The model under review builds one solid part; all positions refer to its coordinate system, in mm. Face numbers are marked on the shaded views. A direction names the side the tool comes from. Round coordinates to 2 decimals unless told otherwise and drop trailing zeros. Order: outer loops, then holes, each group sorted by start corner. A loop starts at its lowest first (then second) coordinate and runs counter-clockwise, first axis right, second up.
from build123d import *

# Parameters (mm, degrees)
F1_DEPTH  = 5
F3_DEPTH  = 80
F4_W      = 16
F4_H      = 15
F4_H_2    = 5
F5_DEPTH  = 20
F7_W      = 16
F7_H      = 15
F7_H_2    = 5
F8_DEPTH  = 20
F10_DEPTH = 16
F11_R     = 6.35
F13_DEPTH = 80
F16_DEPTH = 20
F18_DEPTH = 10


with BuildPart() as f1:
    # F0 (on Top) → F1 (new body)
    with BuildSketch(Plane.XY):
        Polygon((40, 0), (40, 8), (-40, 8), (-40, 0), (-40, -8), (40, -8), align=None)
    extrude(amount=F1_DEPTH)

    # F2 (on face) → F3 (join)
    with BuildSketch(Plane.YZ.offset(40)):
        Polygon((8, 0), (-8, 0), (8, -16), align=None)
    extrude(amount=-F3_DEPTH)

    # F4 (on face) → F5 (join)
    with BuildSketch(Plane.YZ.offset(40)):
        with Locations((0, 12.5)):
            Rectangle(F4_W, F4_H)
        with Locations((0, 2.5)):
            Rectangle(F4_W, F4_H_2)
    extrude(amount=F5_DEPTH)

    # F7 (on face) → F8 (join)
    with BuildSketch(Plane(origin=(-40, 0, 0), x_dir=(0, -1, 0), z_dir=(-1, 0, 0))):
        with Locations((0, 12.5)):
            Rectangle(F7_W, F7_H)
        with Locations((0, 2.5)):
            Rectangle(F7_W, F7_H_2)
    extrude(amount=F8_DEPTH)

    # F9 (on face) + F6 (on face) → F10 (cut)
    with BuildSketch(Plane.XZ.offset(8)):
        with BuildLine():
            ThreePointArc((-44.2724350724, 15.7275649276), (-55.7275649276, 15.7275649276), (-55.7275649276, 4.2724350724))
            Line((-55.7275649276, 4.2724350724), (-50, 10))
            Line((-50, 10), (-44.2724350724, 15.7275649276))
        make_face()
        with BuildLine():
            Line((-50, 10), (-55.7275649276, 4.2724350724))
            ThreePointArc((-55.7275649276, 4.2724350724), (-46.9002641978, 2.5165757867), (-41.9, 10))
            ThreePointArc((-41.9, 10), (-42.5165757867, 13.0997358022), (-44.2724350724, 15.7275649276))
            Line((-44.2724350724, 15.7275649276), (-50, 10))
        make_face()
    with BuildSketch(Plane.XZ.offset(8)):
        with BuildLine():
            ThreePointArc((44.2724350724, 15.7275649276), (44.2724350724, 4.2724350724), (55.7275649276, 4.2724350724))
            Line((55.7275649276, 4.2724350724), (50, 10))
            Line((50, 10), (44.2724350724, 15.7275649276))
        make_face()
        with BuildLine():
            Line((50, 10), (55.7275649276, 4.2724350724))
            ThreePointArc((55.7275649276, 4.2724350724), (57.4834242133, 6.9002641978), (58.1, 10))
            ThreePointArc((58.1, 10), (53.0997358022, 17.4834242133), (44.2724350724, 15.7275649276))
            Line((44.2724350724, 15.7275649276), (50, 10))
        make_face()
    extrude(amount=-F10_DEPTH, mode=Mode.SUBTRACT)

    # F11
    f11_edges = [f1.edges().sort_by_distance(p)[0] for p in [
        (40, 0, 20),
        (60, 0, 20),
        (60, 0, 0),
        (-60, 0, 0),
        (-60, 0, 20),
        (-40, 0, 20),
    ]]
    fillet(f11_edges, radius=F11_R)

    # F12 (on face) → F13 (cut)
    with BuildSketch(Plane.YZ.offset(40)):
        Polygon((8, -16), (8, 0), (-8, 0), align=None)
    extrude(amount=-F13_DEPTH, mode=Mode.SUBTRACT)

    # F14 (on face) + F15 (on face) → F16 (cut)
    with BuildSketch(Plane.XY.offset(20)):
        with BuildLine():
            Line((-50, 0), (-50.6226316309, -1.3646720677))
            ThreePointArc((-50.6226316309, -1.3646720677), (-49.1888118117, -1.2617344107), (-48.5, 0))
            ThreePointArc((-48.5, 0), (-48.7382655893, 0.8111881883), (-49.3773683691, 1.3646720677))
            Line((-49.3773683691, 1.3646720677), (-50, 0))
        make_face()
        with BuildLine():
            ThreePointArc((-49.3773683691, 1.3646720677), (-51.3646720677, 0.6226316309), (-50.6226316309, -1.3646720677))
            Line((-50.6226316309, -1.3646720677), (-50, 0))
            Line((-50, 0), (-49.3773683691, 1.3646720677))
        make_face()
    with BuildSketch(Plane.XY.offset(20)):
        with BuildLine():
            Line((50, 0), (49.3773683691, -1.3646720677))
            ThreePointArc((49.3773683691, -1.3646720677), (50.8111881883, -1.2617344107), (51.5, 0))
            ThreePointArc((51.5, 0), (51.2617344107, 0.8111881883), (50.6226316309, 1.3646720677))
            Line((50.6226316309, 1.3646720677), (50, 0))
        make_face()
        with BuildLine():
            ThreePointArc((50.6226316309, 1.3646720677), (48.6353279323, 0.6226316309), (49.3773683691, -1.3646720677))
            Line((49.3773683691, -1.3646720677), (50, 0))
            Line((50, 0), (50.6226316309, 1.3646720677))
        make_face()
    extrude(amount=-F16_DEPTH, mode=Mode.SUBTRACT)

    # F17 (on face) → F18 (cut)
    with BuildSketch(Plane.XY.offset(5)):
        with BuildLine():
            Line((-22.5, 0), (-24, 0))
            ThreePointArc((-24, 0), (-22.5, -1.5), (-21, 0))
            Line((-21, 0), (-22.5, 0))
        make_face()
        with BuildLine():
            ThreePointArc((-21, 0), (-22.5, 1.5), (-24, 0))
            Line((-24, 0), (-22.5, 0))
            Line((-22.5, 0), (-21, 0))
        make_face()
        with BuildLine():
            Line((22.5, 0), (21, 0))
            ThreePointArc((21, 0), (22.5, -1.5), (24, 0))
            Line((24, 0), (22.5, 0))
        make_face()
        with BuildLine():
            ThreePointArc((24, 0), (22.5, 1.5), (21, 0))
            Line((21, 0), (22.5, 0))
            Line((22.5, 0), (24, 0))
        make_face()
    extrude(amount=-F18_DEPTH, mode=Mode.SUBTRACT)


solid = f1.part
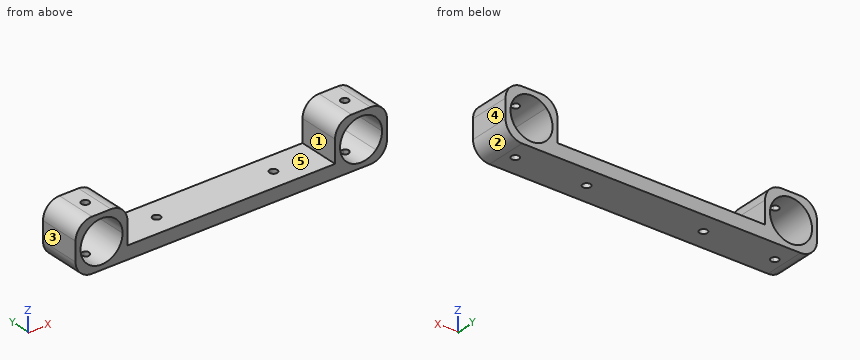
(1) We need section A-A (x = -22.5). Give the boundary of the cut face in (y, z).
(2) Tool access review of the marked faces 4 and 5: name each direction out of +Z, -Z, +X, -X, +Y, -Y from which nothing blocks a thin tool from reaching the whole face with its end or side.
(3) We need section C-C (x = 22). Give the boundary of the cut face in (y, z).
(4) Clearance check with flat-ended pins moving along their axes: P1, Ø1, axis at y = -4.5, z = 5.5, coming from the -X side; P2, Ø12, axis at x = -26, z = 5.5, coming from the -Y side; P3, Ø8, axis at x = -37, y = 5.5, coming from the +Z side; P4, Ø5, axis at x = 31, y = 5, coming from the +Z side. State where each tip first meets the part, or that it passes through.
(5) We need section B-B (y = 4.25). Give the boundary of the cut face in (x, z), and give its area (3 significant figures).
(6) To check wall thickness, follow L1, parallel to X at y = 7.25, z = 9.75; L2, parallel to Y at x = -22.5, z = 2.3; L3, parallel to X at y = 1, z = 15.25. State the ranges of each line that lie inside material, in increasing order.
(7) The part is to be moulded in two halves that separate along X. For the marked faces 1, 2 and 3, say which applies: pulls with the +X half, pulls with the -X half, needs draft (parallel to the pull), parting line crosses it, or undercut.
Verdict:
1. outline: (-8, 0) - (-1.5, 0) - (-1.5, 5) - (-8, 5) - close; (1.5, 0) - (8, 0) - (8, 5) - (1.5, 5) - close
2. face 4: +Z, -Z, +X, +Y, -Y
2. face 5: +Z, +Y, -Y
3. outline: (-8, 0) - (-1.41, 0) - (-1.41, 5) - (-8, 5) - close; (1.41, 0) - (8, 0) - (8, 5) - (1.41, 5) - close
4. P1: stops at x = -59.99
4. P2: stops at y = -8
4. P3: stops at z = 17.07
4. P4: stops at z = 5
5. outline: (-60, 6.35) arc R6.35 ccw to (-53.65, 0) - (53.65, 0) arc R6.35 ccw to (60, 6.35) - (60, 13.65) arc R6.35 ccw to (53.65, 20) - (46.35, 20) arc R6.35 ccw to (40, 13.65) - (40, 5) - (-40, 5) - (-40, 13.65) arc R6.35 ccw to (-46.35, 20) - (-53.65, 20) arc R6.35 ccw to (-60, 13.65) - close; hole circle Ø16.2 at (-50, 10); hole circle Ø16.2 at (50, 10)
5. area: 736 mm2
6. L1: x = -60 to -58.1, -41.9 to -40, 40 to 41.9, 58.1 to 60
6. L2: y = -8 to -1.5, 1.5 to 8
6. L3: x = -59.8 to -56.17, -43.83 to -40.2, 40.2 to 43.83, 56.17 to 59.8
7. face 1: undercut
7. face 2: pulls with the +X half
7. face 3: pulls with the -X half
